Build history of the part. All positions in model axes, mm. A direction names the side the tool comes from. Give positions to 0.01 mm unless a question says otherwise; leave off trailing zeros. Loops run counter-clockwise (first coordinate to the right, second up) from the corner with the lowest first, then second, coordinate; pieces in that order, holes last. Notation, with made-up numbers: (65, 26) -> (87, 26) arc R24 ccw to (87, 64) -> close; hole circle Ø9 at (-19.75, 44). An arc over 180 degrees is marked (long way). One line per question, with ' | ' between items. Start each with the question number.
(1) Slice it at C-C, the plane z = 8. Write the cut outline in (x, y) (3 decimals), then the cut area to 3 significant figures.
(2) Mould opens along X. For faces 6 (the face through (-42.916, -9.881, 0.944)), 7 (the face through (92, 0, 1)), 8 (the face through (195, -25.4, -14)) say: pulls with the +X half, pulls with the -X half, needs draft (parallel to the pull), parting line crosses it, or undercut.
(3) Slice it at B-B, the plane x = 190.5. Write the cut outline in (y, z), then the cut area to 3 significant figures.
(4) 3-axis set-ups, long thin cutter, end or side, ignore diameter. For faces 1 (the face through (42.917, -26.876, -0.871)), 2 (the face through (18.5, -34.925, -18.5)), 3 (the face through (195, 6.35, -14)), 4 (the face through (42.917, 7.826, -0.871)), 5 (the face through (18.5, 15.875, -18.5)): which of +Z, -Z, +X, -X, +Y, -Y reach the whole face in a straight line?
(5) Flat gauge pins, fed straight in: pin 1 Ø5 at (x, y) = (15.5, -6) entering from +Z; pin 2 Ø2 at (x, z) = (104, -33) entering from -Y; pin 3 Ø12 at (y, z) = (0.5, 22) entering from -X. Where does each tip first touch, or does it go through?
(6) Slice it at A-A, the plane y = 10. Write the cut outline in (x, z), then the cut area to 3 significant figures.
(7) Slice it at D-D, the plane y = -3. Write the cut outline in (x, z), then the cut area to 3 significant figures.
(8) Drill centre lines: L1, parallel to X at y = 4.5, z = 3; L2, parallel to X at y = -5, z = -3; L3, parallel to X at y = 3.5, z = 4. Where is each one in solid material? Low to high. Write a range as from..to.
```python
from build123d import *

# Parameters (mm, degrees)
F1_DEPTH = 19.05
F2_DEPTH = 34.925
F3_DEPTH = 25.4
F4_DEPTH = 6.35
F5_DEPTH = 15.875


with BuildPart() as f1:
    # F0 (on Front) → F1 (new body)
    with BuildSketch(Plane.XZ):
        with BuildLine():
            Line((0, -25.4), (0, -42.926))
            Line((0, -42.926), (5.16603969, -42.61400603))
            ThreePointArc((5.16603969, -42.61400603), (32.1278609289, -28.4682635251), (42.926, 0))
            Line((42.926, 0), (25.4, 0))
            ThreePointArc((25.4, 0), (17.9605122421, -17.9605122421), (0, -25.4))
        make_face()
        with BuildLine():
            Line((180.848, 32.004), (5.16603969, 42.61400603))
            ThreePointArc((5.16603969, 42.61400603), (32.1278609289, 28.4682635251), (42.926, 0))
            Line((42.926, 0), (148.844, 0))
            ThreePointArc((148.844, 0), (158.2177545749, 22.6302454251), (180.848, 32.004))
        make_face()
        with BuildLine():
            ThreePointArc((42.926, 0), (32.1278609289, -28.4682635251), (5.16603969, -42.61400603))
            Line((5.16603969, -42.61400603), (180.848, -32.004))
            ThreePointArc((180.848, -32.004), (158.2177545749, -22.6302454251), (148.844, 0))
            Line((148.844, 0), (42.926, 0))
        make_face()
    extrude(amount=F1_DEPTH)

    # F0 (on Front) → F2 (join)
    with BuildSketch(Plane.XZ):
        with BuildLine():
            Line((0, 25.4), (0, 42.926))
            ThreePointArc((0, 42.926), (-42.926, 0), (0, -42.926))
            Line((0, -42.926), (0, -25.4))
            ThreePointArc((0, -25.4), (-25.4, 0), (0, 25.4))
        make_face()
        with BuildLine():
            Line((5.16603969, 42.61400603), (0, 42.926))
            Line((0, 42.926), (0, 25.4))
            ThreePointArc((0, 25.4), (17.9605122421, 17.9605122421), (25.4, 0))
            Line((25.4, 0), (42.926, 0))
            ThreePointArc((42.926, 0), (32.1278609289, 28.4682635251), (5.16603969, 42.61400603))
        make_face()
        with BuildLine():
            Line((0, -25.4), (0, -42.926))
            Line((0, -42.926), (5.16603969, -42.61400603))
            ThreePointArc((5.16603969, -42.61400603), (32.1278609289, -28.4682635251), (42.926, 0))
            Line((42.926, 0), (25.4, 0))
            ThreePointArc((25.4, 0), (17.9605122421, -17.9605122421), (0, -25.4))
        make_face()
    extrude(amount=F2_DEPTH)

    # F0 (on Front) → F3 (join)
    with BuildSketch(Plane.XZ):
        with BuildLine():
            Line((180.848, 17.526), (180.848, 32.004))
            ThreePointArc((180.848, 32.004), (158.2177545749, 22.6302454251), (148.844, 0))
            Line((148.844, 0), (163.322, 0))
            ThreePointArc((163.322, 0), (168.4552465529, 12.3927534471), (180.848, 17.526))
        make_face()
        with BuildLine():
            ThreePointArc((148.844, 0), (158.2177545749, -22.6302454251), (180.848, -32.004))
            Line((180.848, -32.004), (180.848, -17.526))
            ThreePointArc((180.848, -17.526), (168.4552465529, -12.3927534471), (163.322, 0))
            Line((163.322, 0), (148.844, 0))
        make_face()
        with BuildLine():
            ThreePointArc((212.852, 0), (203.4782454251, 22.6302454251), (180.848, 32.004))
            Line((180.848, 32.004), (180.848, 17.526))
            ThreePointArc((180.848, 17.526), (193.2407534471, 12.3927534471), (198.374, 0))
            ThreePointArc((198.374, 0), (193.2407534471, -12.3927534471), (180.848, -17.526))
            Line((180.848, -17.526), (180.848, -32.004))
            ThreePointArc((180.848, -32.004), (203.4782454251, -22.6302454251), (212.852, 0))
        make_face()
    extrude(amount=F3_DEPTH)

    # F0 (on Front) → F4 (join)
    with BuildSketch(Plane.XZ):
        with BuildLine():
            ThreePointArc((212.852, 0), (203.4782454251, 22.6302454251), (180.848, 32.004))
            Line((180.848, 32.004), (180.848, 17.526))
            ThreePointArc((180.848, 17.526), (193.2407534471, 12.3927534471), (198.374, 0))
            ThreePointArc((198.374, 0), (193.2407534471, -12.3927534471), (180.848, -17.526))
            Line((180.848, -17.526), (180.848, -32.004))
            ThreePointArc((180.848, -32.004), (203.4782454251, -22.6302454251), (212.852, 0))
        make_face()
        with BuildLine():
            ThreePointArc((148.844, 0), (158.2177545749, -22.6302454251), (180.848, -32.004))
            Line((180.848, -32.004), (180.848, -17.526))
            ThreePointArc((180.848, -17.526), (168.4552465529, -12.3927534471), (163.322, 0))
            Line((163.322, 0), (148.844, 0))
        make_face()
        with BuildLine():
            Line((180.848, 17.526), (180.848, 32.004))
            ThreePointArc((180.848, 32.004), (158.2177545749, 22.6302454251), (148.844, 0))
            Line((148.844, 0), (163.322, 0))
            ThreePointArc((163.322, 0), (168.4552465529, 12.3927534471), (180.848, 17.526))
        make_face()
    extrude(amount=-F4_DEPTH)

    # F0 (on Front) → F5 (join)
    with BuildSketch(Plane.XZ):
        with BuildLine():
            Line((0, 25.4), (0, 42.926))
            ThreePointArc((0, 42.926), (-42.926, 0), (0, -42.926))
            Line((0, -42.926), (0, -25.4))
            ThreePointArc((0, -25.4), (-25.4, 0), (0, 25.4))
        make_face()
        with BuildLine():
            Line((5.16603969, 42.61400603), (0, 42.926))
            Line((0, 42.926), (0, 25.4))
            ThreePointArc((0, 25.4), (17.9605122421, 17.9605122421), (25.4, 0))
            Line((25.4, 0), (42.926, 0))
            ThreePointArc((42.926, 0), (32.1278609289, 28.4682635251), (5.16603969, 42.61400603))
        make_face()
        with BuildLine():
            Line((0, -25.4), (0, -42.926))
            Line((0, -42.926), (5.16603969, -42.61400603))
            ThreePointArc((5.16603969, -42.61400603), (32.1278609289, -28.4682635251), (42.926, 0))
            Line((42.926, 0), (25.4, 0))
            ThreePointArc((25.4, 0), (17.9605122421, -17.9605122421), (0, -25.4))
        make_face()
    extrude(amount=-F5_DEPTH)


solid = f1.part
```
Final values:
1) outline: (-42.174, -34.925) -> (-24.107, -34.925) -> (-24.107, 15.875) -> (-42.174, 15.875) -> close; (24.107, -34.925) -> (42.174, -34.925) -> (42.174, -19.05) -> (149.86, -19.05) -> (149.86, -25.4) -> (165.254, -25.4) -> (165.254, 6.35) -> (149.86, 6.35) -> (149.86, 0) -> (42.174, 0) -> (42.174, 15.875) -> (24.107, 15.875) -> close; (196.442, -25.4) -> (211.836, -25.4) -> (211.836, 6.35) -> (196.442, 6.35) -> close | area: 4,860 mm2
2) face 6: pulls with the -X half | face 7: undercut | face 8: needs draft
3) outline: (-25.4, -30.51) -> (6.35, -30.51) -> (6.35, -14.63) -> (-25.4, -14.63) -> close; (-25.4, 14.63) -> (6.35, 14.63) -> (6.35, 30.51) -> (-25.4, 30.51) -> close | area: 1,010 mm2
4) face 1: -Y | face 2: +Z, -Z, +X, -X, -Y | face 3: +Z, -Z, +X, +Y | face 4: +Y | face 5: +Z, -Z, +X, -X, +Y
5) pin 1: z = 42.14 | pin 2: y = -19.05 | pin 3: x = -39.83
6) outline: (0, -42.93) -> (5.17, -42.61) arc R42.93 ccw to (5.17, 42.61) -> (0, 42.93) arc R42.93 ccw to start; hole circle Ø50.8 at (0, 0) | area: 3,760 mm2
7) outline: (0, -42.93) -> (180.85, -32) arc R32 ccw to (180.85, 32) -> (0, 42.93) arc R42.93 ccw to start; hole circle Ø50.8 at (0, 0); hole circle Ø35.05 at (180.85, 0) | area: 15,100 mm2
8) L1: -42.82..-25.22, 25.22..42.82, 148.98..163.58, 198.12..212.71 | L2: -42.82..-25.22, 25.22..163.58, 198.12..212.71 | L3: -42.74..-25.08, 25.08..42.74, 149.09..163.78, 197.91..212.6
